from build123d import *

# Parameters (mm, degrees)
SKETCH2_W           = 18.7
SKETCH2_H           = 20
BOSS_EXTRUDE1_DEPTH = 25.4
SKETCH3_W           = 6.35
SKETCH3_H           = 7.3
SKETCH3_H_2         = 3.175
CUT_EXTRUDE1_DEPTH  = 21
SKETCH5_W           = 3.175
SKETCH5_H           = 25.4
BOSS_EXTRUDE2_DEPTH = 20
SKETCH6_W           = 10
SKETCH6_H           = 10.125
CUT_EXTRUDE2_DEPTH  = 16.825
SKETCH7_W           = 3
SKETCH7_H           = 3.5
CUT_EXTRUDE3_DEPTH  = 10
SKETCH8_W           = 22
SKETCH8_H           = 10.125
CUT_EXTRUDE4_DEPTH  = 19
SKETCH9_W           = 2.175
SKETCH9_H           = 14.925
BOSS_EXTRUDE3_DEPTH = 25.05
SKETCH10_W          = 1.825
SKETCH10_H          = 7.8
CUT_EXTRUDE5_DEPTH  = 4.5


with BuildPart() as part:
    # Sketch2 → Boss-Extrude1 (new body)
    with BuildSketch(Plane(origin=(0, 0, 0), x_dir=(1, 0, 0), z_dir=(0, 1, 0))):
        Rectangle(SKETCH2_W, SKETCH2_H)
    extrude(amount=BOSS_EXTRUDE1_DEPTH)

    # Sketch3 → Cut-Extrude1 (cut, through all)
    with BuildSketch(Plane(origin=(0, 0, -10), x_dir=(-1, 0, 0), z_dir=(0, 0, -1))):
        with Locations((0, 21.75)):
            Rectangle(SKETCH3_W, SKETCH3_H)
        with Locations((0, 16.5125)):
            Rectangle(SKETCH3_W, SKETCH3_H_2)
    extrude(amount=-CUT_EXTRUDE1_DEPTH, mode=Mode.SUBTRACT)

    # Sketch5 → Boss-Extrude2 (add)
    with BuildSketch(Plane(origin=(0, 0, -10), x_dir=(-1, 0, 0), z_dir=(0, 0, -1))):
        with Locations((-10.9375, 12.7)):
            Rectangle(SKETCH5_W, SKETCH5_H)
        with Locations((10.9375, 12.7)):
            Rectangle(SKETCH5_W, SKETCH5_H)
    extrude(amount=-BOSS_EXTRUDE2_DEPTH)

    # Sketch6 → Cut-Extrude2 (cut)
    with BuildSketch(Plane(origin=(0, 0, -10), x_dir=(-1, 0, 0), z_dir=(0, 0, -1))):
        Polygon((5, 22.225), (5, 10.125), (5, 0), (9.35, 0), (9.35, 22.225), align=None)
        with Locations((0, 5.0625)):
            Rectangle(SKETCH6_W, SKETCH6_H)
        Polygon((-5, 22.225), (-9.35, 22.225), (-9.35, 0), (-5, 0), (-5, 10.125), align=None)
    extrude(amount=-CUT_EXTRUDE2_DEPTH, mode=Mode.SUBTRACT)

    # Sketch7 → Cut-Extrude3 (cut)
    with BuildSketch(Plane(origin=(5, 0, 0), x_dir=(0, 0, -1), z_dir=(1, 0, 0))):
        with Locations((-4.825, 19.725)):
            Rectangle(SKETCH7_W, SKETCH7_H)
    extrude(amount=-CUT_EXTRUDE3_DEPTH, mode=Mode.SUBTRACT)

    # Sketch8 → Cut-Extrude4 (cut)
    with BuildSketch(Plane(origin=(0, 0, -10), x_dir=(-1, 0, 0), z_dir=(0, 0, -1))):
        with Locations((0, 5.0625)):
            Rectangle(SKETCH8_W, SKETCH8_H)
    extrude(amount=-CUT_EXTRUDE4_DEPTH, mode=Mode.SUBTRACT)

    # Sketch9 → Boss-Extrude3 (add)
    with BuildSketch(Plane(origin=(12.525, 0, 0), x_dir=(0, 0, -1), z_dir=(1, 0, 0))):
        with Locations((-11.0875, 7.4625)):
            Rectangle(SKETCH9_W, SKETCH9_H)
    extrude(amount=-BOSS_EXTRUDE3_DEPTH)

    # Sketch10 → Cut-Extrude5 (cut)
    with BuildSketch(Plane(origin=(0, 0, 2.325), x_dir=(-1, 0, 0), z_dir=(0, 0, -1))):
        with Locations((-4.0875, 21.5)):
            Rectangle(SKETCH10_W, SKETCH10_H)
        with Locations((4.0875, 21.5)):
            Rectangle(SKETCH10_W, SKETCH10_H)
    extrude(amount=-CUT_EXTRUDE5_DEPTH, mode=Mode.SUBTRACT)


solid = part.part
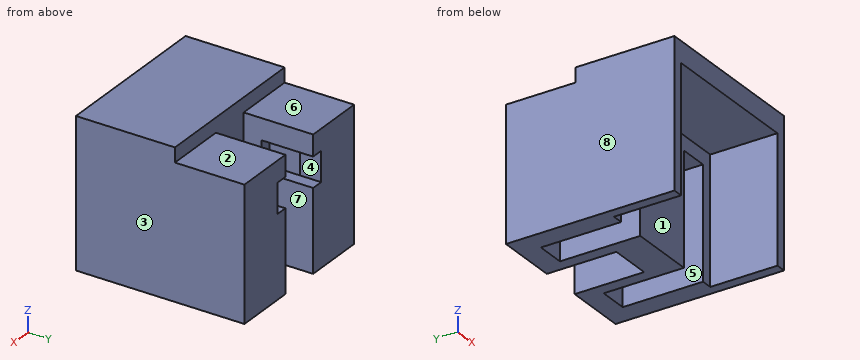
The listing builds one solid part. Answer for the finished solid, in the listing's coordinates (mm). Face numbers are marked on the shaded views. A direction names the side the tool comes from. Round coordinates to 2 decimals unless told otherwise and drop trailing zeros. Order: outer loops, then holes, each group sorted by start corner. A loop starts at its lowest first (then second) coordinate and runs counter-clockwise, first axis right, second up. Notation, with made-up numbers: (29.5, -9) - (39.5, -9) arc R13 cw to (39.5, 14) - close; hole circle Ø6 at (12.5, 25.25). An arc over 180 degrees is marked (long way). Write item = value, one per line. Start each with the question number.
1) For the marked faces 4, 5, 6, 7 and 8, determine the directions among +Z, -Z, +X, -X, +Y, -Y from which every point of the face is accessible in a straight line to the end or side of a thin tool.
2) Section D-D, the plane y = 12.75 is taken. Write down the section's boundary in (x, z) (3 decimals).
3) Straight lines are drawn through the part: L1, parallel to X at y = 13, z = -2 (3 decimals); L2, parallel to X at y = 20.75, z = -4.5 (3 decimals); L3, parallel to X at y = 21.5, z = 9 (3 decimals). For each, find the intervals that lie inside material, in ascending order.
4) Section A-A, the plane y = 15.75 is taken. Write down the section's boundary in (x, z) (3 decimals), plus the area to 3 significant figures.
5) For a pull along X with two mould halves and no side action, classify the marked faces 1, 2 and 3 as released by +X, released by -X, zero draft, split by the parting line, or undercut.
6) Section B-B, the plane z = 3.75 is taken. Write down the section's boundary in (x, y) (3 decimals), plus the area to 3 significant figures.
7) Section C-C, the plane x = 9.75 is taken. Write down the section's boundary in (y, z) (3 decimals), plus the area to 3 significant figures.
8) Given pin 1 (0.9 mm diameter, centred on x = -4, z = 5.5, fed in from +Y); pin 2 (3 mm diameter, centred on x = 5.5, y = 6, fed in from -Z); pin 3 (7.5 mm diameter, centred on x = -7.5, y = 22.5, fed in from +Z), each flat-ended and moving along its own axis, determine where each tip first touches the part or whether it passes through.
Results list:
q1.face_4 = +Y
q1.face_5 = -Z, -Y
q1.face_6 = +Z, +X, -X, +Y
q1.face_7 = +Z, -Z, +Y
q1.face_8 = +Z, -Z, -X, +Y, -Y
q2.outline = (-12.525, -10) - (-9.35, -10) - (-9.35, 6.825) - (-5, 6.825) - (-5, -10) - (5, -10) - (5, 6.825) - (9.35, 6.825) - (9.35, -10) - (12.525, -10) - (12.525, 12.175) - (-12.525, 12.175) - close
q3.L1 = -12.525 to -9.35, -5 to 5, 9.35 to 12.525
q3.L2 = -12.525 to -9.35, -5 to -3.175, 3.175 to 5, 9.35 to 12.525
q3.L3 = -12.525 to -3.175, 3.175 to 12.525
q4.outline = (-12.525, -10) - (-9.35, -10) - (-9.35, 6.825) - (-5, 6.825) - (-5, -10) - (-3.175, -10) - (-3.175, 10) - (-12.525, 10) - close; (3.175, -10) - (5, -10) - (5, 6.825) - (9.35, 6.825) - (9.35, -10) - (12.525, -10) - (12.525, 10) - (3.175, 10) - close
q4.area = 228 mm^2
q5.face_1 = undercut
q5.face_2 = zero draft
q5.face_3 = released by +X
q6.outline = (-12.525, 0) - (-11, 0) - (-11, 10.125) - (-9.35, 10.125) - (-9.35, 22.225) - (-5, 22.225) - (-5, 25.4) - (-12.525, 25.4) - close; (-5, 10.125) - (5, 10.125) - (5, 17.6) - (3.175, 17.6) - (3.175, 14.925) - (-3.175, 14.925) - (-3.175, 17.6) - (-5, 17.6) - close; (5, 22.225) - (9.35, 22.225) - (9.35, 10.125) - (11, 10.125) - (11, 0) - (12.525, 0) - (12.525, 25.4) - (5, 25.4) - close
q6.area = 213 mm^2
q7.outline = (0, 9) - (10.125, 9) - (10.125, -10) - (25.4, -10) - (25.4, 10) - (14.925, 10) - (14.925, 12.175) - (0, 12.175) - close
q7.area = 348 mm^2
q8.pin_1 = 17.6
q8.pin_2 = 9
q8.pin_3 = 10
